from build123d import *

# Parameters (mm, degrees)
SKETCH1_R           = 13.335
SKETCH1_R_2         = 10.4648
BOSS_EXTRUDE1_DEPTH = 187.325
SKETCH1_2_R         = 10.4648
BOSS_EXTRUDE2_DEPTH = 4.7625
SKETCH3_R           = 3.175
CUT_EXTRUDE1_DEPTH  = 14.351


with BuildPart() as part:
    # Sketch1 → Boss-Extrude1 (new body)
    with BuildSketch(Plane(origin=(0, 0, 0), x_dir=(1, 0, 0), z_dir=(0, 1, 0))):
        Circle(SKETCH1_R)
        Circle(SKETCH1_R_2, mode=Mode.SUBTRACT)
    extrude(amount=BOSS_EXTRUDE1_DEPTH)

    # Sketch1<2> → Boss-Extrude2 (add)
    with BuildSketch(Plane(origin=(0, 0, 0), x_dir=(1, 0, 0), z_dir=(0, 1, 0))):
        Circle(SKETCH1_2_R)
    extrude(amount=BOSS_EXTRUDE2_DEPTH)

    # Sketch3 → Cut-Extrude1 (cut)
    with BuildSketch(Plane(origin=(13.335, 0, 0), x_dir=(0, 0, -1), z_dir=(1, 0, 0))):
        with Locations((0, 7.9375)):
            Circle(SKETCH3_R)
    extrude(amount=-CUT_EXTRUDE1_DEPTH, mode=Mode.SUBTRACT)


solid = part.part
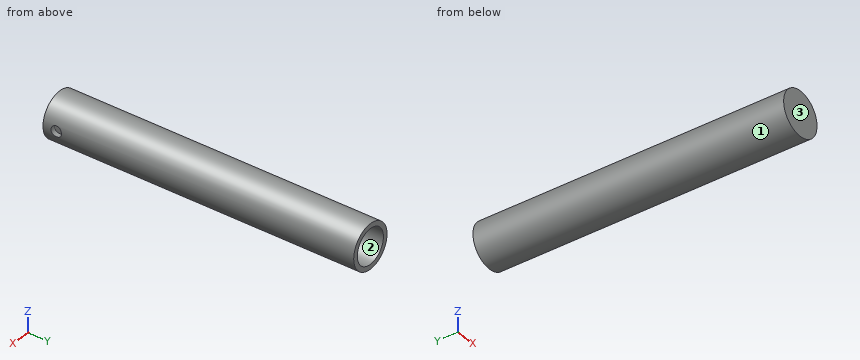
Geometry check sheet. Reference: the model listing, model coordinates, mm. Face numbers are marked on the shaded views. Round coordinates to 2 decimals unless told otherwise and drop trailing zeros. Write each loop counter-clockwise with the first axis right and the second up, starting at its lowest first coordinate (ties: lowest second). Pieces come first, ordered by that corner, then holes. Notation, with made-up numbers: (-37, -15.5) -> (-7, -15.5) arc R20 ccw to (-7, -10.5) -> close; hole circle Ø9 at (22, 13.5). An arc over 180 degrees is marked (long way). One line per item, written item: value. Start each with the question number.
(1) Go/stop test with flat-tipped pins: pin 1 Ø6 at (y, z) = (69, -6.5) entering from -X; pin 2 Ø1.5 at (x, y) = (5.5, 133.5) entering from -Z; pin 3 Ø3 at (x, z) = (-8, 1.5) entering from +Y. Record where each tip stops, or that it passes through.
(2) Draft check along Z on the marked faces 1, 2 and 3. Enter one of: +Z half, -Z half, draft (parallel to the pull), parting line (faces both ways), or undercut.
(3) Cross-section at C-C, the plane x = 6. Record the cut outline in (y, z) (1 decimal).
(4) Cross-section at B-B, the plane z = -8.5. Record the cut outline in (x, y) (1 decimal).
(5) Scan lines: line 1 (X direction, y = 128, z = 0) (3 decimals); line 2 (Y direction, x = 10.75, z = 0) (1 decimal). Record each from-to range of solid material in increasing order. Write a range as [from, to].
(6) Cross-section at A-A, the plane y = 121. Record the cut outline in (x, z) (3 decimals).
Answer:
1. pin 1: x = -12.87
1. pin 2: z = -12.46
1. pin 3: y = 4.76
2. face 1: parting line
2. face 2: undercut
2. face 3: draft
3. outline: (0, -11.9) -> (187.3, -11.9) -> (187.3, -8.6) -> (4.8, -8.6) -> (4.8, 8.6) -> (187.3, 8.6) -> (187.3, 11.9) -> (0, 11.9) -> close
4. outline: (-10.3, 0) -> (10.3, 0) -> (10.3, 187.3) -> (6.1, 187.3) -> (6.1, 4.8) -> (-6.1, 4.8) -> (-6.1, 187.3) -> (-10.3, 187.3) -> close
5. line 1: [-13.335, -10.465], [10.465, 13.335]
5. line 2: [0, 4.8], [11.1, 187.3]
6. outline: circle Ø26.67 at (0, 0); hole circle Ø20.93 at (0, 0)
